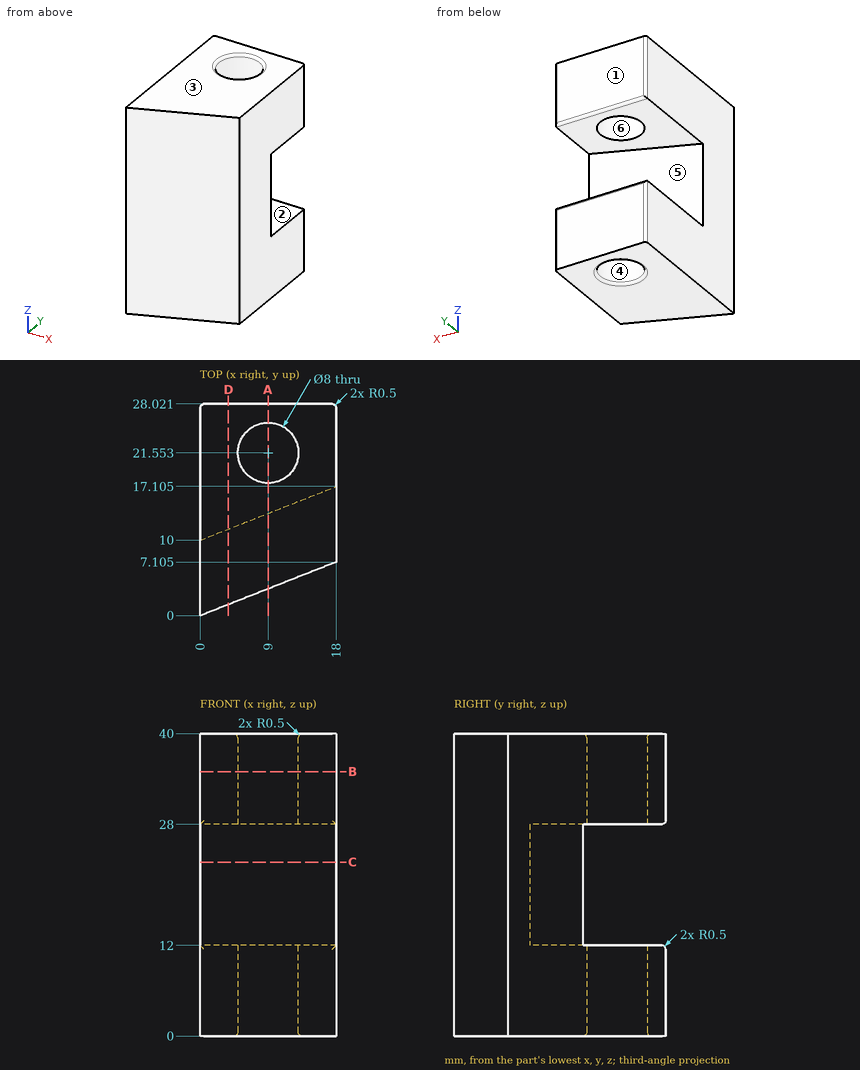
Answer from the drawing. Dimensions are ordinates in mm from the lowest x, y and z of the part. A direction names the side the tool comes from. Give positions to 0.01 mm unless a question says otherwise; leave off trailing zeros. Order: outer loops, then holes, each group sorted by start corner. A loop starts at its lowest first (then second) coordinate and runs counter-clockwise, first axis right, second up. Notation, with made-up numbers: (8.5, -35.5) - (12.5, -35.5) arc R22 ccw to (12.5, 2.5) - close; hole circle Ø3 at (40, -17.75). An arc over 180 degrees is marked (long way). Use one line per item in the form item = value.
1) Find section C-C on z = 23. Determine the outline of the cut face in (x, y) (1 decimal).
Verdict:
outline = (0, 0) - (18, 7.1) - (18, 17.1) - (0, 10) - close
2) The mould has two halves that part along Y. Classify the marked faces 3, 4, 5 and 6: released by +Y, released by -Y, zero draft, split by the parting line, or undercut.
Verdict:
face_3 = zero draft
face_4 = undercut
face_5 = released by +Y
face_6 = undercut
3) Consider probe 1 along Z at (x, y) = (16, 17); probe 2 along Y at (x, z) = (9, 4); probe 3 along X at (y, z) = (21, 3.5). Determine where each line is inside the solid, lowest interval first. Write a range as [from, to].
Verdict:
probe_1 = [0, 12], [28, 40]
probe_2 = [3.55, 17.55], [25.55, 28.02]
probe_3 = [0, 5.04], [12.96, 18]
4) Find section A-A on x = 9. Determine the outline of the cut face in (y, z).
Verdict:
outline = (3.55, 0) - (17.05, 0) arc R0.5 ccw to (17.55, 0.5) - (17.55, 12) - (13.55, 12) - (13.55, 28) - (17.55, 28) - (17.55, 39.5) arc R0.5 ccw to (17.05, 40) - (3.55, 40) - close; (25.55, 0.5) arc R0.5 ccw to (26.05, 0) - (28.02, 0) - (28.02, 11.5) arc R0.5 ccw to (27.52, 12) - (25.55, 12) - close; (25.55, 28) - (27.52, 28) arc R0.5 ccw to (28.02, 28.5) - (28.02, 40) - (26.05, 40) arc R0.5 ccw to (25.55, 39.5) - close
5) Each of these flat-tipped pins is pushed along its axis until it touches: pin 1 (6 mm diameter, centred on x = 11.5, z = 17.5, fed in from +Y); pin 2 (4 mm diameter, centred on x = 2.5, z = 9.5, fed in from -Y); pin 3 (5 mm diameter, centred on x = 9, y = 21.55, fed in from -Z). Where does it stop, or does it pass through?
Verdict:
pin_1 = 15.72
pin_2 = 0.2
pin_3 = through
6) For the marked faces 1 and 2, determine the directions among +Z, -Z, +X, -X, +Y, -Y from which every point of the face is accessible in a straight line to the end or side of a thin tool.
Verdict:
face_1 = +Z, -Z, +X, -X, +Y
face_2 = -X, +Y
7) Find section B-B on z = 35. Determine the outline of the cut face in (x, y) (1 decimal).
Verdict:
outline = (0, 0) - (18, 7.1) - (18, 27.5) arc R0.5 ccw to (17.5, 28) - (0.5, 28) arc R0.5 ccw to (0, 27.5) - close; hole circle Ø8 at (9, 21.6)
8) Find section D-D on x = 3.75. Determine the outline of the cut face in (y, z).
Verdict:
outline = (1.48, 0) - (28.02, 0) - (28.02, 11.5) arc R0.5 ccw to (27.52, 12) - (11.48, 12) - (11.48, 28) - (27.52, 28) arc R0.5 ccw to (28.02, 28.5) - (28.02, 40) - (1.48, 40) - close
